Geometry: final body of the model. Coordinates: model frame, mm. Face numbers are marked on the shaded views. A direction names the side the tool comes from. Round coordinates to 2 decimals unless told otherwise and drop trailing zeros. Order: outer loops, then holes, each group sorted by start corner. A loop starts at its lowest first (then second) coordinate and runs counter-clockwise, first axis right, second up. Notation, with made-up numbers: (68.5, 44.25) -> (81.5, 44.25) arc R15 cw to (81.5, 57.25) -> close; hole circle Ø4 at (-25, -25). An arc over 180 degrees is marked (long way). Put each result on its own line as item: value.
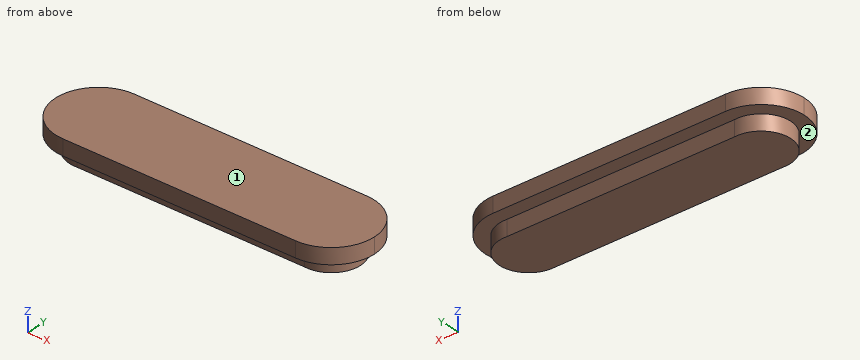
```python
from build123d import *

# Parameters (mm, degrees)
F1_DEPTH = 2
F3_DEPTH = 2


with BuildPart() as f1:
    # F0 (on Top) → F1 (new body)
    with BuildSketch(Plane.XY):
        with BuildLine():
            ThreePointArc((19.640177, 0.03416), (18.008268, 3.884303), (14.140506, 5.474007))
            Line((14.140506, 5.474007), (-15.859494, 5.474007))
            ThreePointArc((-15.859494, 5.474007), (-19.748581, 3.863094), (-21.359494, -0.025993))
            ThreePointArc((-21.359494, -0.025993), (-19.748581, -3.915081), (-15.859494, -5.525993))
            Line((-15.859494, -5.525993), (14.140506, -5.525993))
            ThreePointArc((14.140506, -5.525993), (18.050803, -3.893755), (19.640177, 0.03416))
        make_face()
    extrude(amount=F1_DEPTH)

    # F2 (on face) → F3 (join)
    with BuildSketch(Plane(origin=(0, 0, 0), x_dir=(1, 0, 0), z_dir=(0, 0, -1))):
        with BuildLine():
            Line((13.778, 3.760071), (-15.496988, 3.760071))
            ThreePointArc((-15.496988, 3.760071), (-19.592193, 0.025993), (-15.496988, -3.708084))
            Line((-15.496988, -3.708084), (13.778, -3.708084))
            ThreePointArc((13.778, -3.708084), (17.873205, 0.025993), (13.778, 3.760071))
        make_face()
    extrude(amount=F3_DEPTH)


solid = f1.part
```
1. Cut plane D-D on y = 4.5. Return loops of the section in (x, z).
Ans:
outline: (-18.98, 0) -> (17.27, 0) -> (17.27, 2) -> (-18.98, 2) -> close
2. Contact query for flat-ended pins moving along their axis: P1, Ø1, axis at x = -4, z = -1, coming from the -Y side; P2, Ø2, axis at y = -3.5, z = 0, coming from the +X side. Output: stop coordinate, or through.
Ans:
P1: y = -3.76
P2: x = 19.05
3. Cut plane C-C on y = 0.75. Return loops of the section in (x, z).
Ans:
outline: (-21.3, 0) -> (-19.51, 0) -> (-19.51, -2) -> (17.79, -2) -> (17.79, 0) -> (19.59, 0) -> (19.59, 2) -> (-21.3, 2) -> close
4. Cut plane B-B on z = 0.35. Return loops of the section in (x, y).
Ans:
outline: (-21.36, -0.03) arc R5.5 ccw to (-15.86, -5.53) -> (14.14, -5.53) arc R5.5 ccw to (19.64, 0.03) arc R5.5 ccw to (14.14, 5.47) -> (-15.86, 5.47) arc R5.5 ccw to start
5. Cut plane A-A on x = -11. Return loops of the section in (y, z).
Ans:
outline: (-5.53, 0) -> (-3.76, 0) -> (-3.76, -2) -> (3.71, -2) -> (3.71, 0) -> (5.47, 0) -> (5.47, 2) -> (-5.53, 2) -> close
6. Set-up query: the marked faces 1 and 2. Return all of +Z, -Z, +X, -X, +Y, -Y with unobstructed straight access to the full face (end or side cutting, diameter ignored); none if empty.
Ans:
face 1: +Z, +X, -X, +Y, -Y
face 2: -Z
7. Material intervals for probe 1 along Z at (x, y) = (18, -2.75); probe 2 along Y at (x, z) = (14, -1.4); probe 3 along X at (y, z) = (-0.5, 0.6), sorted ascending.
Ans:
probe 1: 0 to 2
probe 2: -3.77 to 3.72
probe 3: -21.34 to 19.62
